Print and shaded views of the part. All mm, measured from the part's lowest x, y and z. A direction names the side the tool comes from. Coordinates: 2 decimals unless noted, no trailing zeros. Order: outer loops, then holes, each group sorted by start corner. A loop starts at its lowest first (then second) coordinate and runs counter-clockwise, first axis right, second up. Notation, with made-up numbers: (72, 71.25) -> (115, 71.25) arc R15 ccw to (115, 87.25) -> close; hole circle Ø1 at (8, -26.5). An arc over 180 degrees is marked (long way). Write item = value, one per line. Start each with the question number.
Q1. Wall check: line 1 (Z direction, x = 38.1, y = 11.25) (1 decimal); line 2 (Y direction, x = 38.1, z = 34) (1 decimal); line 3 (Z direction, x = 33, y = 38). Give the ranges that are in metal, low to high. Write a range as from..to.
Q2. Cut at C-C, the plane y = 7.5. Give the number of separate pieces and of enclosed holes in the cut face, plus the area to 3 significant figures.
Q3. Cut at B-B, the plane z = 12.7. List the corners of the cut face in (x, y) (1 decimal), plus the area to 3 significant figures.
Q4. 3-axis set-ups, long thin cutter, end or side, ignore diameter. For the marked faces 1, 2, 3 and 4: which of +Z, -Z, +X, -X, +Y, -Y reach the whole face in a straight line?
Q5. Cut at A-A, the plane x = 12.7. List the corners of the cut face in (y, z) (1 decimal), plus the area to 3 significant figures.
Q6. Flat gauge pins, fed straight in: pin 1 (24.5 mm diameter, centred on y = 17, z = 66.5, fed in from +X); pin 2 (12 mm diameter, centred on x = 42.5, z = 63, fed in from +Y); pin 3 (10 mm diameter, centred on x = 33.5, y = 45.5, fed in from +Z); pin 4 (12 mm diameter, centred on y = 25.5, z = 24, fed in from +X). Where does each tip first touch, or does it go through?
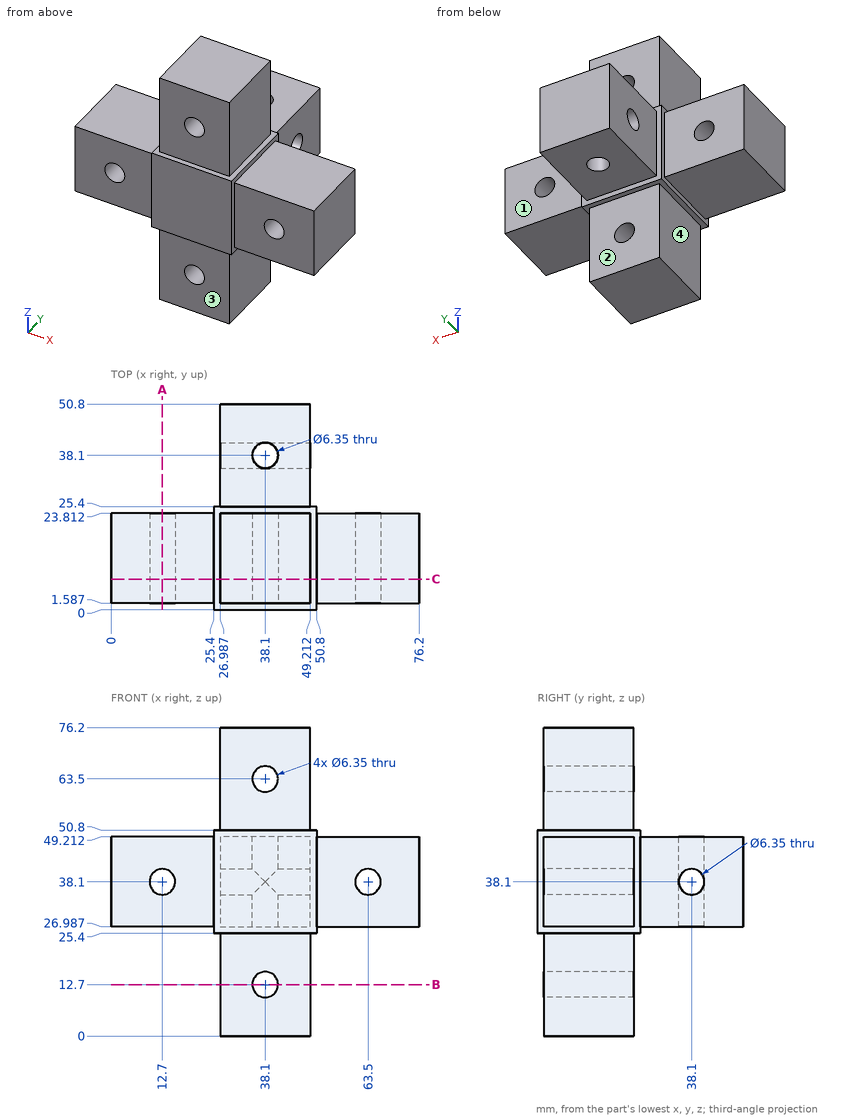
Here are the results:
q1.line_1 = 0..9.5, 15.9..60.3, 66.7..76.2
q1.line_2 = 0..34.9, 41.3..50.8
q1.line_3 = 26.99..34.93, 41.27..49.21
q2.separate_pieces = 1
q2.enclosed_holes = 4
q2.area = 2,780 mm²
q3.outline = (27, 1.6) -> (34.9, 1.6) -> (34.9, 23.8) -> (27, 23.8) -> close; (41.3, 1.6) -> (49.2, 1.6) -> (49.2, 23.8) -> (41.3, 23.8) -> close
q3.area = 353 mm²
q4.face_1 = +Z, -Z, +X, +Y
q4.face_2 = -Z, +X, -X, +Y
q4.face_3 = -Z, +X, -X, -Y
q4.face_4 = -Z, -X, +Y, -Y
q5.outline = (1.6, 27) -> (23.8, 27) -> (23.8, 34.9) -> (1.6, 34.9) -> close; (1.6, 41.3) -> (23.8, 41.3) -> (23.8, 49.2) -> (1.6, 49.2) -> close
q5.area = 353 mm²
q6.pin_1 = 49.21
q6.pin_2 = 23.81
q6.pin_3 = 49.21
q6.pin_4 = 76.2
